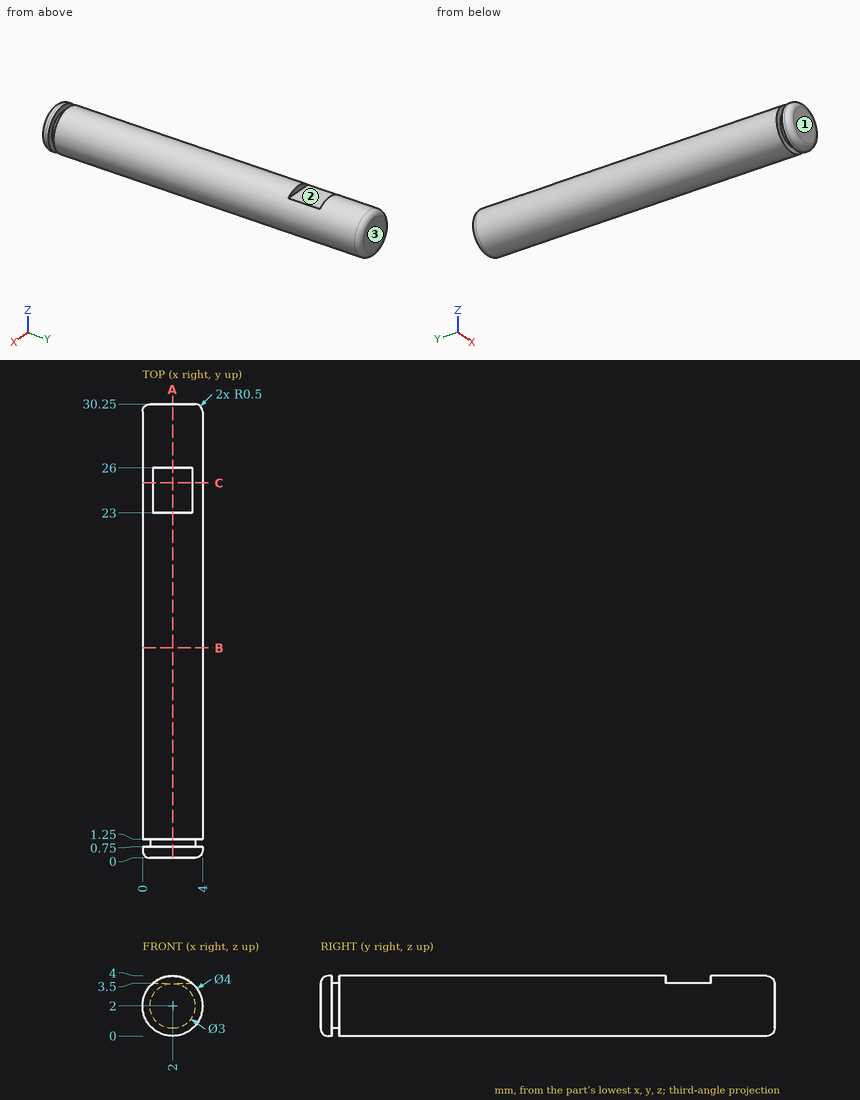
For this review, use the dimensioned drawing (mm, ordinates from the lowest corner) and the shaded views. Give positions to 0.01 mm unless a question says otherwise; leave off trailing zeros. Order: outer loops, then holes, each group sorted by start corner. A loop starts at its lowest first (then second) coordinate and runs counter-clockwise, first axis right, second up. Notation, with made-up numbers: (57.5, 54.5) - (84.5, 54.5) arc R23 ccw to (84.5, 63.5) - close; hole circle Ø10 at (30.25, 89). An arc over 180 degrees is marked (long way). Use a Markdown table: item, result. Add a question column.
(1) Add section B-B on y = 14. Give the boundary of the cut face in (x, z), then the cut area to 3 significant figures.
(2) Wall thickness on probe 1 along Y at (x, z) = (3.75, 1.6); probe 2 along X at (y, z) = (14, 2.1); probe 3 along Y at (x, z) = (3.5, 1.4): over which ranges is each line inside the solid? List them lowest first. Write a range as [from, to].
(3) Mouldability with a two-part tool opening along Y and no side actions: class the marked faces 1, 2 and 3 as +Y half, -Y half, draft (parallel to the pull), parting line (faces both ways), or undercut.
(4) Clearance check with flat-ended pins moving along their axes: P1, Ø0.8, axis at x = 1.5, y = 24.5, coming from the +Z side; P2, Ø2, axis at x = 1.5, z = 2.5, coming from the -Y side. State where each tip first meets the part, or that it passes through.
(5) Add section C-C on y = 25. Give the boundary of the cut face in (x, z).
(6) Add section A-A on x = 2. Give the boundary of the cut face in (y, z).
Report:
| question | item | result |
|---|---|---|
| 1 | outline | circle Ø4 at (2, 2) |
| 1 | area | 12.6 mm² |
| 2 | probe 1 | y = [0.1, 0.75], [1.25, 30.15] |
| 2 | probe 2 | x = [0, 4] |
| 2 | probe 3 | y = [0.01, 0.75], [1.25, 30.24] |
| 3 | face 1 | -Y half |
| 3 | face 2 | undercut |
| 3 | face 3 | +Y half |
| 4 | P1 | stops at z = 3.5 |
| 4 | P2 | stops at y = 0 |
| 5 | outline | (0.68, 3.5) arc R2 ccw (long way) to (3.32, 3.5) - close |
| 6 | outline | (0, 0.5) arc R0.5 ccw to (0.5, 0) - (0.75, 0) - (0.75, 0.5) - (1.25, 0.5) - (1.25, 0) - (29.75, 0) arc R0.5 ccw to (30.25, 0.5) - (30.25, 3.5) arc R0.5 ccw to (29.75, 4) - (26, 4) - (26, 3.5) - (23, 3.5) - (23, 4) - (1.25, 4) - (1.25, 3.5) - (0.75, 3.5) - (0.75, 4) - (0.5, 4) arc R0.5 ccw to (0, 3.5) - close |
